Check sheet for the drawn part. Datum: minimum x, y, z corner. Units: mm. Give positions to 0.01 mm unless a question says otherwise; leave off trailing zeros. Loops run counter-clockwise (first coordinate to the right, second up) from the corner with the lowest first, then second, coordinate; pieces in that order, holes last.
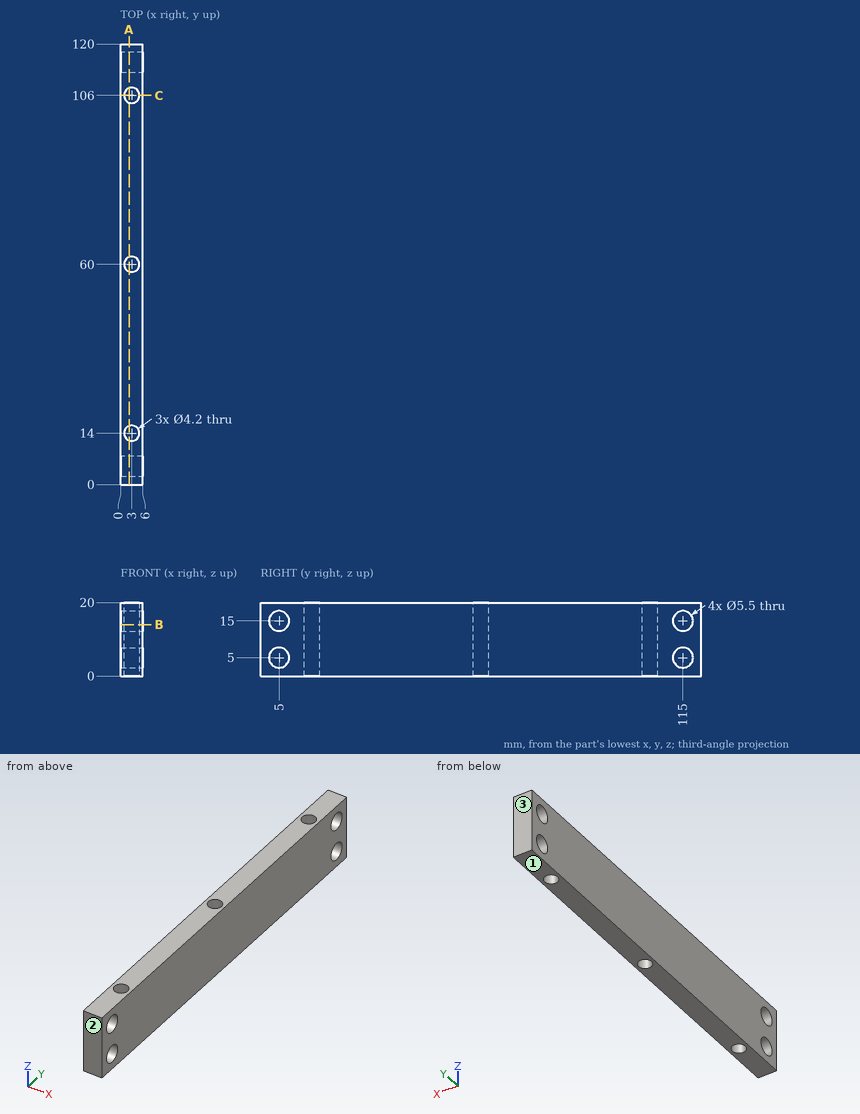
(1) Material ranges on line 1 (Z direction, x = 4.55, y = 5); line 2 (Y direction, x = 3, z = 9.25); line 3 (Y direction, x = 0.4, z = 14.75), recorded low to high.
(2) Section check C-C on y = 106. Record the boundary of the cut face in (x, z).
(3) Release check for a two-part mould opening along Y. For the marked faces 1, 2 and 3 record: pulls with the +Y half, pulls with the -Y half, needs draft (parallel to the pull), parting line crosses it, or undercut.
(4) Section check A-A on x = 2.3. Record the boundary of the cut face in (y, z).
(5) Section check B-B on z = 14. Record the boundary of the cut face in (x, y), plus the area to 3 significant figures.
(6) Gauge pin test, flat end, axial feed: pin 1 Ø6.5 at (y, z) = (5, 15) entering from -X. Record the tip position at first contact, or that the pin passes through.
Computed values:
1. line 1: z = 0 to 2.25, 7.75 to 12.25, 17.75 to 20
1. line 2: y = 0 to 11.9, 16.1 to 57.9, 62.1 to 103.9, 108.1 to 120
1. line 3: y = 0 to 2.26, 7.74 to 112.26, 117.74 to 120
2. outline: (0, 0) - (0.9, 0) - (0.9, 20) - (0, 20) - close; (5.1, 0) - (6, 0) - (6, 20) - (5.1, 20) - close
3. face 1: needs draft
3. face 2: pulls with the -Y half
3. face 3: pulls with the +Y half
4. outline: (0, 0) - (12.02, 0) - (12.02, 20) - (0, 20) - close; (15.98, 0) - (58.02, 0) - (58.02, 20) - (15.98, 20) - close; (61.98, 0) - (104.02, 0) - (104.02, 20) - (61.98, 20) - close; (107.98, 0) - (120, 0) - (120, 20) - (107.98, 20) - close; hole circle Ø5.5 at (5, 5); hole circle Ø5.5 at (5, 15); hole circle Ø5.5 at (115, 5); hole circle Ø5.5 at (115, 15)
5. outline: (0, 0) - (6, 0) - (6, 2.44) - (0, 2.44) - close; (0, 7.56) - (6, 7.56) - (6, 112.44) - (0, 112.44) - close; (0, 117.56) - (6, 117.56) - (6, 120) - (0, 120) - close; hole circle Ø4.2 at (3, 14); hole circle Ø4.2 at (3, 60); hole circle Ø4.2 at (3, 106)
5. area: 617 mm2
6. pin 1: stops at x = 0
